Read the model definition and answer for the solid it produces. Units are mm, in the model's axes. A direction names the side the tool comes from. Coordinates: 2 decimals unless noted, no trailing zeros. Write each loop counter-clockwise with the first axis right and the second up, starting at its lowest first coordinate (ties: lowest second). Pieces come first, ordered by that corner, then holes. Notation, with made-up numbers: (-39, 59.25) -> (1, 59.25) arc R18 ccw to (1, 67.25) -> close; hole circle Ø7 at (89.25, 4). An arc over 180 degrees is marked (long way). Answer as a JSON object with one key per item and string values. Group by question number.
(1) Find section C-C (z = -17.5). Give the vertices of the cut face in (x, y).
(2) Find section B-B (y = -1.5). Count the separate pieces of the cut face and the enclosed holes in it, then the cut area to 3 significant figures.
(3) Straight lines are drawn through the part: L1, parallel to Y at x = -6.3, z = -4.8 (3 decimals); L2, parallel to X at y = 0.5, z = -14; L3, parallel to Z at x = 5, y = -0.5. For each, find the intervals that lie inside material, in ascending order.
(4) For a pull along Y with two mould halves and no side action, classify faces 1 (the face through (0, 5, 7)), 2 (the face through (3.653, 3.967, 6.726)), 3 (the face through (-5.572, 0.713, -14.535)), 4 (the face through (4.76, -2.75, 6.73)) as +Y half, -Y half, draft (parallel to the pull), parting line (faces both ways), or undercut.
(5) Find section A-A (z = -4.8). Give the vertices of the cut face in (x, y) (3 decimals), then the cut area to 4 significant figures.
(6) Flat-ended cylindrical pins translate along their axes: P1, Ø4.5, axis at y = -2, z = -17, coming from the +X side; P2, Ø1.3, axis at x = -0.5, y = -2, coming from the -Z side; P3, Ø4, axis at y = 4, z = 6.5, coming from the +X side; P4, Ø3, axis at y = 0, z = -16.8, coming from the +X side. Find the tip coordinate at first contact, or state that the pin passes through.
(7) Which of the six approach directions +Z, -Z, +X, -X, +Y, -Y give full straight-line access (tool end or side, diameter ignored) to faces 5 (the face through (6.8, 3.9, 4)), 6 (the face through (0, 0, 0)), 7 (the face through (3, 0, 5.4))?
from build123d import *
from build123d.topology import SkipClean

# Parameters (mm, degrees)
ESQUISSE1_W             = 14.2
ESQUISSE1_H             = 9
BOSS_EXTRU_3_DEPTH      = 4
ESQUISSE4_W             = 3.1
ESQUISSE4_H             = 9
BOSS_EXTRU_4_DEPTH      = 23.5
ESQUISSE5_R             = 2.375
ENL_V_MAT_EXTRU_2_DEPTH = 28.823371471
ESQUISSE6_R             = 7.5
BOSS_EXTRU_5_DEPTH      = 1
CONG_1_R                = 0.5
EXTRU_MINCE1_DEPTH      = 3.5
ESQUISSE10_R            = 0.5
ESQUISSE10_W            = 4.21226809
ESQUISSE10_H            = 2.7


with BuildPart() as part:
    # Esquisse1 → Boss.-Extru.3 (new body)
    with BuildSketch(Plane.XY):
        Rectangle(ESQUISSE1_W, ESQUISSE1_H)
    extrude(amount=BOSS_EXTRU_3_DEPTH)

    # Esquisse4 → Boss.-Extru.4 (add)
    with BuildSketch(Plane(origin=(0, 0, 0), x_dir=(-1, 0, 0), z_dir=(0, 0, -1))):
        with Locations((5.55, 0)):
            Rectangle(ESQUISSE4_W, ESQUISSE4_H)
        with Locations((-5.55, 0)):
            Rectangle(ESQUISSE4_W, ESQUISSE4_H)
    extrude(amount=BOSS_EXTRU_4_DEPTH)

    # Esquisse5 → Enlèv. mat.-Extru.2 (cut, through all)
    with BuildSketch(Plane.ZY.offset(7.1)):
        with Locations((-16.8, 0)):
            Circle(ESQUISSE5_R)
        with Locations((-4.8, 0)):
            Circle(ESQUISSE5_R)
    extrude(amount=-ENL_V_MAT_EXTRU_2_DEPTH, mode=Mode.SUBTRACT)

    # Esquisse6 → Boss.-Extru.5 (add)
    with BuildSketch(Plane.XY.offset(4)):
        with Locations(Location((0, 0, 0), (0, 0, 161.203094965))):
            Circle(ESQUISSE6_R)
    extrude(amount=BOSS_EXTRU_5_DEPTH)

    # Congé1
    # the kernel refuses this fillet: 0.5 mm, written as the material it adds along each edge
    with BuildSketch(Plane(origin=(-7.1, -3.666609195, 4), x_dir=(0, 0, -1), z_dir=(0, 1, 0))) as cong_1_piece_1_section:
        with BuildLine():
            CenterArc((CONG_1_R, CONG_1_R), CONG_1_R, 180, 90)
            Line((0, CONG_1_R), (0, 0))
            Line((0, 0), (CONG_1_R, 0))
        make_face()
    cong_1_piece_1 = extrude(amount=7.333218389, mode=Mode.PRIVATE)
    cong_1_piece_1 = cong_1_piece_1 & Plane(origin=(0, 0, 3.878104255), x_dir=(-0.946666666666828, 0.3222145592953816, 0), z_dir=(0, 0, -1)) * Cylinder(7.5, 17, mode=Mode.PRIVATE)
    add(cong_1_piece_1)
    with BuildSketch(Plane(origin=(7.25, -4.5, 4), x_dir=(0, 0, -1), z_dir=(-1, 0, 0))) as cong_1_piece_2_section:
        with BuildLine():
            CenterArc((CONG_1_R, CONG_1_R), CONG_1_R, 180, 90)
            Line((0, CONG_1_R), (0, 0))
            Line((0, 0), (CONG_1_R, 0))
        make_face()
    cong_1_piece_2 = extrude(amount=14.5, mode=Mode.PRIVATE)
    cong_1_piece_2 = cong_1_piece_2 & Plane(origin=(0, 0, 3.887627019), x_dir=(-0.946666666666828, 0.3222145592953816, 0), z_dir=(0, 0, -1)) * Cylinder(7.5, 32, mode=Mode.PRIVATE)
    add(cong_1_piece_2)
    with BuildSketch(Plane(origin=(7.1, 3.666609195, 4), x_dir=(0, 0, -1), z_dir=(0, -1, 0))) as cong_1_piece_3_section:
        with BuildLine():
            CenterArc((CONG_1_R, CONG_1_R), CONG_1_R, 180, 90)
            Line((0, CONG_1_R), (0, 0))
            Line((0, 0), (CONG_1_R, 0))
        make_face()
    cong_1_piece_3 = extrude(amount=7.333218389, mode=Mode.PRIVATE)
    cong_1_piece_3 = cong_1_piece_3 & Plane(origin=(0, 0, 3.87809802), x_dir=(-0.946666666666828, 0.3222145592953816, 0), z_dir=(0, 0, -1)) * Cylinder(7.5, 17, mode=Mode.PRIVATE)
    add(cong_1_piece_3)
    with BuildSketch(Plane(origin=(-7.25, 4.5, 4), x_dir=(0, 0, -1), z_dir=(1, 0, 0))) as cong_1_piece_4_section:
        with BuildLine():
            CenterArc((CONG_1_R, CONG_1_R), CONG_1_R, 180, 90)
            Line((0, CONG_1_R), (0, 0))
            Line((0, 0), (CONG_1_R, 0))
        make_face()
    cong_1_piece_4 = extrude(amount=14.5, mode=Mode.PRIVATE)
    cong_1_piece_4 = cong_1_piece_4 & Plane(origin=(0, 0, 3.88762702), x_dir=(-0.946666666666828, 0.3222145592953816, 0), z_dir=(0, 0, -1)) * Cylinder(7.5, 32, mode=Mode.PRIVATE)
    add(cong_1_piece_4)

    # Esquisse8 → Extru.-Mince1 (add)
    with SkipClean():  # the faces are left unmerged after this step: merging them gives an invalid solid
        with BuildSketch(Plane.XY.offset(5)):
            with BuildLine():
                ThreePointArc((5.080001443, 5.517570601), (7.414056481, 1.132151268), (6.495190528, -3.75))
                Line((6.495190528, -3.75), (0.08660254, -0.05))
                ThreePointArc((0.08660254, -0.05), (0.098854086, 0.01509535), (0.067733353, 0.073567608))
                Line((0.067733353, 0.073567608), (5.080001443, 5.517570601))
            make_face()
            with BuildLine():
                ThreePointArc((2.238355587, -7.158195601), (-2.726556481, -6.986836892), (-6.495190528, -3.75))
                Line((-6.495190528, -3.75), (-0.08660254, -0.05))
                ThreePointArc((-0.08660254, -0.05), (-0.036354086, -0.093157825), (0.029844741, -0.095442608))
                Line((0.029844741, -0.095442608), (2.238355587, -7.158195601))
            make_face()
            with BuildLine():
                ThreePointArc((-7.318357029, 1.640625), (-4.6875, 5.854685623), (0, 7.5))
                Line((0, 7.5), (0, 0.1))
                ThreePointArc((0, 0.1), (-0.0625, 0.078062475), (-0.097578094, 0.021875))
                Line((-0.097578094, 0.021875), (-7.318357029, 1.640625))
            make_face()
        extrude(amount=EXTRU_MINCE1_DEPTH)
    add(part.part.scale(1), mode=Mode.REPLACE)  # the faces are merged on a copy

    # Esquisse10 → Enlèvement de matière-Révolution1 (revolve, cut)
    with BuildSketch(Plane(origin=(0, 0, 0), x_dir=(1, 0, 0), z_dir=(0, 1, 0)), mode=Mode.PRIVATE) as enl_vement_de_mati_re_r_volution1_sk:
        with Locations((-4, -6.75)):
            Circle(ESQUISSE10_R)
        with Locations((2.573867398, -6.75)):
            Rectangle(ESQUISSE10_W, ESQUISSE10_H)
    revolve(enl_vement_de_mati_re_r_volution1_sk.sketch.rotate(Axis((0, 0, 2.6), (0, 0, 1)), 347.364374907), axis=Axis((0, 0, 2.6), (0, 0, 1)), mode=Mode.SUBTRACT)


solid = part.part
Results below:
{
 "1": {"outline": "(-7.1, -4.5) -> (-4, -4.5) -> (-4, -2.27) -> (-7.1, -2.27) -> close; (-7.1, 2.27) -> (-4, 2.27) -> (-4, 4.5) -> (-7.1, 4.5) -> close; (4, -4.5) -> (7.1, -4.5) -> (7.1, -2.27) -> (4, -2.27) -> close; (4, 2.27) -> (7.1, 2.27) -> (7.1, 4.5) -> (4, 4.5) -> close"},
 "2": {"separate pieces": "6", "enclosed holes": "0", "area": "186 mm2"},
 "3": {"L1": "y = -4.5 to -2.375, 2.375 to 4.5", "L2": "x = -7.1 to -4, 4 to 7.1", "L3": "z = -23.5 to -19.12, -14.48 to -7.12, -2.48 to 8.5"},
 "4": {"face 1": "draft", "face 2": "+Y half", "face 3": "undercut", "face 4": "undercut"},
 "5": {"outline": "(-7.1, -4.5) -> (-4, -4.5) -> (-4, -2.375) -> (-7.1, -2.375) -> close; (-7.1, 2.375) -> (-4, 2.375) -> (-4, 4.5) -> (-7.1, 4.5) -> close; (4, -4.5) -> (7.1, -4.5) -> (7.1, -2.375) -> (4, -2.375) -> close; (4, 2.375) -> (7.1, 2.375) -> (7.1, 4.5) -> (4, 4.5) -> close", "area": "26.35 mm2"},
 "6": {"P1": "stops at x = 7.1", "P2": "stops at z = 0", "P3": "stops at x = 7.23", "P4": "passes through"},
 "7": {"face 5": "+Z, +X, +Y", "face 6": "-Z, +Y, -Y", "face 7": "none"}
}
